Work out the finished part from the listing and answer in its coordinate system (mm). Face numbers are marked on the shaded views. A direction names the side the tool comes from. Coordinates: 2 decimals unless noted, no trailing zeros. Order: outer loops, then holes, each group sorted by start corner. A loop starts at its lowest first (then second) coordinate and runs counter-clockwise, first axis right, second up. Notation, with made-up numbers: (0, 31) -> (39, 31) arc R14 cw to (39, 49) -> close; hole circle Ø1 at (24, -2). An arc over 180 degrees is marked (long way). Answer as CSV lines item,"result". Start each with the question number.
Item 1: Each of these flat-tipped pins is pushed along its axis until it touches: pin 1 Ø6 at (x, z) = (100.5, -51) entering from +Y; pin 2 Ø6 at (x, z) = (55, -85.5) entering from -Y; pin 3 Ø19 at (x, z) = (49.5, -101.5) entering from +Y; pin 4 Ø5 at (x, z) = (-70.5, 60.75) entering from -Y. Where does it stop, or does it pass through?
Item 2: Straight lines are drawn through the part: L1, parallel to X at y = -45, z = -18; L2, parallel to X at y = -13.5, z = 54.5; L3, parallel to Z at x = -11.5, y = 19.5. For each, find the intervals that lie inside material, in ascending order.
Item 3: Section A-A (y = -9) is taken. Write down the section's boundary in (x, z).
Item 4: Section B-B (z = -86.5) is taken. Write down the section's boundary in (x, y), then the cut area to 3 significant figures.
Item 5: Which of the six approach directions +Z, -Z, +X, -X, +Y, -Y give full straight-line access (tool end or side, diameter ignored) to the marked faces 4, 5 and 6?
Item 6: Section C-C (x = 111.5) is taken. Write down the section's boundary in (y, z).
Item 7: For a pull along Z with two mould halves and no side action, classify the marked faces 1, 2 and 3 as pulls with the +Z half, pulls with the -Z half, needs draft (parallel to the pull), parting line crosses it, or undercut.
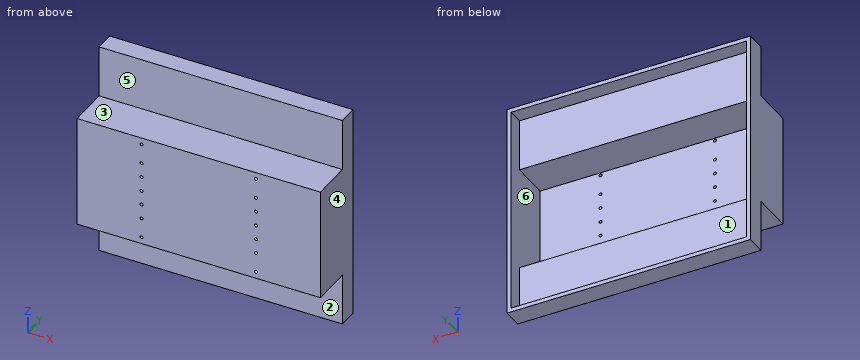
```python
from build123d import *

# Parameters (mm, degrees)
BOSS_EXTRUDE1_DEPTH = 150
SHELL1_START        = -42
SHELL1_OUTLINE_W    = 290
SHELL1_OUTLINE_H    = 128
SHELL1_DEPTH        = 61
SHELL1_START_2      = 5
SHELL1_2_OUTLINE_W  = 290
SHELL1_2_OUTLINE_H  = 64
SHELL1_2_DEPTH      = 14
SKETCH2_R           = 1.85
CUT_EXTRUDE2_DEPTH  = 207.613165118
SKETCH3_W           = 290
SKETCH3_H           = 256
CUT_EXTRUDE3_DEPTH  = 5


# Read off the part's stored shape, not the designer's step: Shell1
with BuildPart() as part:
    # Sketch1 → Boss-Extrude1 (new, symmetric)
    with BuildSketch(Plane(origin=(0, 0, 0), x_dir=(0, 0, -1), z_dir=(1, 0, 0))):
        Polygon((-69, 0), (-133, 0), (-133, 24), (133, 24), (133, 0), (69, 0), (69, -50), (-69, -50), align=None)
    extrude(amount=BOSS_EXTRUDE1_DEPTH, both=True)

    # Shell1 outline → Shell1 (cut)
    with BuildSketch(Plane(origin=(0, 0, 0), x_dir=(1, 0, 0), z_dir=(0, 1, 0)).offset(SHELL1_START)):
        Rectangle(SHELL1_OUTLINE_W, SHELL1_OUTLINE_H)
    extrude(amount=SHELL1_DEPTH, mode=Mode.SUBTRACT)

    # Shell1 2 outline → Shell1 2 (cut)
    with BuildSketch(Plane(origin=(0, 0, 0), x_dir=(1, 0, 0), z_dir=(0, 1, 0)).offset(SHELL1_START_2)):
        with Locations((0, 96)):
            Rectangle(SHELL1_2_OUTLINE_W, SHELL1_2_OUTLINE_H)
        with Locations((0, -96)):
            Rectangle(SHELL1_2_OUTLINE_W, SHELL1_2_OUTLINE_H)
    extrude(amount=SHELL1_2_DEPTH, mode=Mode.SUBTRACT)

    # Sketch2 → Cut-Extrude2 (cut, through all)
    with BuildSketch(Plane(origin=(0, 0, 0), x_dir=(1, 0, 0), z_dir=(0, 1, 0))):
        with Locations(Location((70.5, 0, 0), (0, 0, 270))):
            Circle(SKETCH2_R)
        with Locations(Location((70.5, 18, 0), (0, 0, 270))):
            Circle(SKETCH2_R)
        with Locations(Location((70.5, 36, 0), (0, 0, 270))):
            Circle(SKETCH2_R)
        with Locations(Location((70.5, -18, 0), (0, 0, 270))):
            Circle(SKETCH2_R)
        with Locations(Location((70.5, -36, 0), (0, 0, 270))):
            Circle(SKETCH2_R)
        with Locations(Location((70.5, -60.75, 0), (0, 0, 270))):
            Circle(SKETCH2_R)
        with Locations(Location((70.5, 60.75, 0), (0, 0, 270))):
            Circle(SKETCH2_R)
        with Locations(Location((-70.5, -60.75, 0), (0, 0, 270))):
            Circle(SKETCH2_R)
        with Locations(Location((-70.5, -36, 0), (0, 0, 270))):
            Circle(SKETCH2_R)
        with Locations(Location((-70.5, -18, 0), (0, 0, 270))):
            Circle(SKETCH2_R)
        with Locations(Location((-70.5, 0, 0), (0, 0, 270))):
            Circle(SKETCH2_R)
        with Locations(Location((-70.5, 18, 0), (0, 0, 270))):
            Circle(SKETCH2_R)
        with Locations(Location((-70.5, 36, 0), (0, 0, 270))):
            Circle(SKETCH2_R)
        with Locations(Location((-70.5, 60.75, 0), (0, 0, 270))):
            Circle(SKETCH2_R)
    extrude(amount=-CUT_EXTRUDE2_DEPTH, mode=Mode.SUBTRACT)

    # Sketch3 → Cut-Extrude3 (cut)
    with BuildSketch(Plane(origin=(0, 24, 0), x_dir=(1, 0, 0), z_dir=(0, 1, 0))):
        Rectangle(SKETCH3_W, SKETCH3_H)
    extrude(amount=-CUT_EXTRUDE3_DEPTH, mode=Mode.SUBTRACT)


solid = part.part
```
Checked values:
1,pin 1,"stops at y = -42"
1,pin 2,"stops at y = 0"
1,pin 3,"stops at y = 5"
1,pin 4,"stops at y = -50"
2,L1,"x = -150 to -72.35, -68.65 to 68.65, 72.35 to 150"
2,L2,"x = -150 to -145, 145 to 150"
2,L3,"z = -133 to -128, 128 to 133"
3,outline,"(-150, -69) -> (150, -69) -> (150, 69) -> (-150, 69) -> close; hole (-145, -64) -> (145, -64) -> (145, 64) -> (-145, 64) -> close"
4,outline,"(-150, 0) -> (150, 0) -> (150, 24) -> (145, 24) -> (145, 5) -> (-145, 5) -> (-145, 24) -> (-150, 24) -> close"
4,area,"1,690 mm^2"
5,face 4,"+Z, -Z, +X, +Y, -Y"
5,face 5,"+Z, +X, -X, -Y"
5,face 6,"+Y"
6,outline,"(-50, -69) -> (0, -69) -> (0, -133) -> (24, -133) -> (24, -128) -> (5, -128) -> (5, -64) -> (-42, -64) -> (-42, 64) -> (5, 64) -> (5, 128) -> (24, 128) -> (24, 133) -> (0, 133) -> (0, 69) -> (-50, 69) -> close"
7,face 1,"undercut"
7,face 2,"needs draft"
7,face 3,"pulls with the +Z half"
